```python
from build123d import *

# Parameters (mm, degrees)
F_3_4_16_TAPPED_HOLE1_D     = 17.4625
F_3_4_16_TAPPED_HOLE1_DEPTH = 12.5222
F_3_4_16_TAPPED_HOLE1_TIP   = 8.73125
SKETCH9_R                   = 4.7625
THRU_HOLE_DEPTH             = 62.384040094
WRENCH_FLATS_7_8_DEPTH      = 12.7
BREAK_ALL_EDGES_SIZE        = 0.254
F_8_32_TAPPED_HOLE1_D       = 3.4544
F_8_32_TAPPED_HOLE1_DEPTH   = 4.3688


with BuildPart() as part:
    # Sketch1 → Revolve1 (revolve)
    with BuildSketch(Plane(origin=(0, 0, 0), x_dir=(0, 0, -1), z_dir=(1, 0, 0))):
        Polygon((0, 0), (-12.7, 0), (-12.7, -30.1625), (-19.05, -30.1625), (-19.05, -31.7373), (-6.35, -31.7373), (-6.35, -34.5313), (-19.05, -34.5313), (-19.05, -36.1061), (-6.35, -36.1061), (-6.35, -55.1561), (0, -55.1561), align=None)
    revolve(axis=Axis((0, 0, 0), (0, -1, 0)))

    # Sketch5 → 1/8 NPT Tapped Hole1 (revolve, cut)
    with BuildSketch(Plane(origin=(12.7, -21.2725, 0), x_dir=(0, 0, -1), z_dir=(0, 1, 0))):
        Polygon((0, 0), (0, 14.166668714), (4.2164, 11.6332), (4.2164, 6.9342), (4.936185566, 6.9342), (5.1438048, 0), align=None)
    revolve(axis=Axis((19.05, -21.2725, 0), (-1, 0, 0)), mode=Mode.SUBTRACT)

    # 3/4-16 Tapped Hole1
    with Locations(Plane(origin=(0, 0, 0), x_dir=(-1, 0, 0), z_dir=(0, 1, 0))):
        with Locations((0, 0)):
            Hole(F_3_4_16_TAPPED_HOLE1_D / 2, depth=F_3_4_16_TAPPED_HOLE1_DEPTH)
            with Locations((0, 0, -(F_3_4_16_TAPPED_HOLE1_DEPTH + F_3_4_16_TAPPED_HOLE1_TIP / 2))):  # 90° drill point
                Cone(0, F_3_4_16_TAPPED_HOLE1_D / 2, F_3_4_16_TAPPED_HOLE1_TIP, mode=Mode.SUBTRACT)

    # Sketch9 → Thru hole (cut, through all)
    with BuildSketch(Plane.XZ.offset(55.1561)):
        with Locations(Location((0, 0, 0), (0, 0, 270))):
            Circle(SKETCH9_R)
    extrude(amount=-THRU_HOLE_DEPTH, mode=Mode.SUBTRACT)

    # Sketch10 → Wrench flats 7/8" (cut, symmetric)
    with BuildSketch(Plane(origin=(0, 0, 0), x_dir=(0, 0, -1), z_dir=(1, 0, 0))):
        with BuildLine():
            Line((-12.7, -14.2875), (-12.5095, -14.2875))
            ThreePointArc((-12.5095, -14.2875), (-11.431869265, -14.733869265), (-10.9855, -15.8115))
            Line((-10.9855, -15.8115), (-10.9855, -25.4635))
            ThreePointArc((-10.9855, -25.4635), (-11.431869265, -26.541130735), (-12.5095, -26.9875))
            Line((-12.5095, -26.9875), (-12.7, -26.9875))
            Line((-12.7, -26.9875), (-12.7, -14.2875))
        make_face()
        with BuildLine():
            Line((10.9855, -15.8115), (10.9855, -25.4635))
            ThreePointArc((10.9855, -25.4635), (11.431869265, -26.541130735), (12.5095, -26.9875))
            Line((12.5095, -26.9875), (12.7, -26.9875))
            Line((12.7, -26.9875), (12.7, -14.2875))
            Line((12.7, -14.2875), (12.5095, -14.2875))
            ThreePointArc((12.5095, -14.2875), (11.431869265, -14.733869265), (10.9855, -15.8115))
        make_face()
    extrude(amount=WRENCH_FLATS_7_8_DEPTH, both=True, mode=Mode.SUBTRACT)

    # Break all edges
    break_all_edges_edges = [part.edges().sort_by_distance(p)[0] for p in [
        (0, -34.5313, -19.05),
        (0, -36.1061, -19.05),
        (0, -55.1561, -6.35),
        (0, -55.1561, 4.7625),
        (0, 0, -12.7),
        (0, -30.1625, -19.05),
        (0, -31.7373, -19.05),
    ]]
    chamfer(break_all_edges_edges, length=BREAK_ALL_EDGES_SIZE)

    # #8-32 Tapped Hole1
    with Locations(Plane(origin=(0, -30.1625, 0), x_dir=(-1, 0, 0), z_dir=(0, 1, 0))):
        with Locations((0, 15.875)):
            Hole(F_8_32_TAPPED_HOLE1_D / 2, depth=F_8_32_TAPPED_HOLE1_DEPTH)


solid = part.part
```
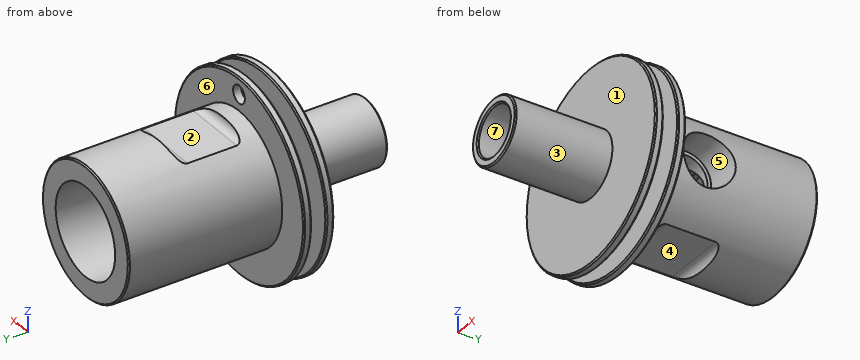
Source: CAD feature listing. Evaluate the final solid. Frame: model axes, mm. Face numbers are marked on the shaded views. A direction names the side the tool comes from. Coordinates: 2 decimals unless noted, no trailing zeros. Loops run counter-clockwise (first coordinate to the right, second up) from the corner with the lowest first, then second, coordinate; pieces in that order, holes last. Notation, with made-up numbers: M -1,33 L 51,33 A21 cw 51,58 Z; hole C -4,14 d9. An arc over 180 degrees is marked long. Use CSV: the item, a comma, the result in double quotes.
(1) Draft query along Y for the marked faces 1, 2, 3 and 4. Return one class per face: pulls with the +Y half, pulls with the -Y half, needs draft (parallel to the pull), parting line crosses it, or undercut.
Answers follow:
face 1,"pulls with the -Y half"
face 2,"undercut"
face 3,"needs draft"
face 4,"undercut"
(2) Cut plane B-B on z = 0. Give the number of separate pieces and of enclosed holes in the cut face, and give its area (3 significant figures).
Answers follow:
separate pieces,"3"
enclosed holes,"0"
area,"444 mm²"
(3) Cut plane A-A on y = -5.5. Return loops of the section in (x, z), and give its area (3 significant figures).
Answers follow:
outline,"C 0,0 d25.4; hole C 0,0 d17.46"
area,"267 mm²"
(4) Contact query for flat-ended pins moving along their axis: pin 1 (1.5 mm diameter, centred on y = -22, z = 6, fed in from +X); pin 2 (3 mm diameter, centred on y = -19.5, z = 0.5, fed in from +X); pin 3 (12 mm diameter, centred on x = 15, z = -13, fed in from -Y). Output: stop coordinate, or through.
Answers follow:
pin 1,"x = 11.56"
pin 2,"x = -4.32"
pin 3,"y = -36.11"
(5) Reachability of the marked faces 5, 6 and 7 from +Z, -Z, +X, -X, +Y, -Y: full face, straight path, thin tool, end or side. Return the list, or none.
Answers follow:
face 5,"+X"
face 6,"+Y"
face 7,"+Y, -Y"
(6) Line query: line 1 (Z direction, x = 0, y = -28); line 2 (Z direction, x = 0, y = -4); line 3 (Y direction, x = 15.5, z = -0.5). Output: solid intervals per line, ascending. Write a range as [from, to].
Answers follow:
line 1,"[-12.7, -4.76], [4.76, 12.7]"
line 2,"[-12.7, -8.73], [8.73, 12.7]"
line 3,"[-36.11, -34.53], [-31.74, -30.16]"
